Design review of the part built by this model. Coordinates are the model's own, in mm. A direction names the side the tool comes from. Give positions to 0.01 mm unless a question says otherwise; leave off trailing zeros. Loops run counter-clockwise (first coordinate to the right, second up) from the corner with the lowest first, then second, coordinate; pieces in that order, holes last.
from build123d import *

# Parameters (mm, degrees)
SKETCH1_R           = 3.175
BOSS_EXTRUDE1_DEPTH = 6
SKETCH2_R           = 4.25
BOSS_EXTRUDE2_DEPTH = 44
SKETCH3_R           = 3.175
BOSS_EXTRUDE3_DEPTH = 6
FILLET1_R           = 1


with BuildPart() as part:
    # Sketch1 → Boss-Extrude1 (new body)
    with BuildSketch(Plane.XY):
        Circle(SKETCH1_R)
    extrude(amount=BOSS_EXTRUDE1_DEPTH)

    # Sketch2 → Boss-Extrude2 (add)
    with BuildSketch(Plane(origin=(0, 0, 0), x_dir=(-1, 0, 0), z_dir=(0, 0, -1))):
        Circle(SKETCH2_R)
    extrude(amount=BOSS_EXTRUDE2_DEPTH)

    # Sketch3 → Boss-Extrude3 (add)
    with BuildSketch(Plane(origin=(0, 0, -44), x_dir=(-1, 0, 0), z_dir=(0, 0, -1))):
        Circle(SKETCH3_R)
    extrude(amount=BOSS_EXTRUDE3_DEPTH)

    # Fillet1
    fillet1_edges = [part.edges().sort_by_distance(p)[0] for p in [
        (3.175, 0, -50),
        (-3.175, 0, 6),
    ]]
    fillet(fillet1_edges, radius=FILLET1_R)


solid = part.part
Q1. Tool access review of faces 1 (the face through (-0.69, -3.1, 2.46)), 2 (the face through (-2.285, 3.584, -21.692)), 3 (the face through (0.69, -3.1, -46.46)): name each direction out of +Z, -Z, +X, -X, +Y, -Y from which nothing blocks a thin tool from reaching the whole face with its end or side.
Results:
face 1: +Z
face 2: +Z, -Z
face 3: -Z
Q2. Insertion check: pin 1 (3 mm diameter, centred on x = -3, z = -25, fed in from -Y). The pin has a flat end and moves straight along its axis. Give the tip position at first contact, or say it passes through.
Results:
pin 1: stops at y = -3.98
Q3. Wall thickness on line 1 (Z direction, x = -3.5, y = 1); line 2 (Z direction, x = 0, y = -2.25); line 3 (Y direction, x = 2, z = -23): over which ranges is each line inside the solid? List them lowest first.
Results:
line 1: z = -44 to 0
line 2: z = -50 to 6
line 3: y = -3.75 to 3.75
Q4. Take a section at A-A (y = 0). Give the boundary of the cut face in (x, z) (3 decimals), plus the area to 3 significant figures.
Results:
outline: (-4.25, -44) - (-3.175, -44) - (-3.175, -49) arc R1 ccw to (-2.175, -50) - (2.175, -50) arc R1 ccw to (3.175, -49) - (3.175, -44) - (4.25, -44) - (4.25, 0) - (3.175, 0) - (3.175, 5) arc R1 ccw to (2.175, 6) - (-2.175, 6) arc R1 ccw to (-3.175, 5) - (-3.175, 0) - (-4.25, 0) - close
area: 449 mm2
Q5. Take a section at C-C (z = -42). Give the boundary of the cut face in (x, y).
Results:
outline: circle Ø8.5 at (0, 0)
